Input: dimensioned drawing with shaded views. Units: mm. Origin: part minimum x, y, z. A direction names the side the tool comes from. Give positions to 0.01 mm unless a question says otherwise; leave off trailing zeros. Write each loop counter-clockwise with the first axis right and the second up, starting at its lowest first coordinate (ties: lowest second). Pieces come first, ordered by that corner, then holes. Notation, with made-up numbers: (39.25, -25.75) -> (56.25, -25.75) arc R24 cw to (56.25, -1.75) -> close; hole circle Ø10 at (70, 1.25). An arc over 180 degrees is marked (long way). Return JSON: item names as keys, results as strings. Group by question number.
Item 1: Pin query (flat end, axial travel): P1, Ø1.5, axis at x = 47.5, y = 790.5, coming from the +Z side; P2, Ø1.5, axis at y = 250.5, z = 168.5, coming from the +X side; P3, Ø8, axis at x = 73.5, y = 418.5, coming from the +Z side. Return the tip coordinate at first contact, or that it passes through.
Item 2: Section D-D, the plane z = 89. Return loops of the section in (x, y), then the cut area to 3 significant figures.
Item 3: Line query: line 1 (Z direction, x = 50, y = 231.5); line 2 (X direction, y = 511, z = 130.5) (1 decimal); line 3 (X direction, y = 529, z = 137.5). Output: solid intervals per line, ascending. Write a range as [from, to].
Item 4: Section A-A, the plane x = 50. Return loops of the section in (y, z).
Item 5: Section B-B, the plane z = 150. Return loops of the section in (x, y), then the cut area to 3 significant figures.
Item 6: Section C-C, the plane y = 500.5. Return loops of the section in (x, z), then the cut area to 3 significant figures.
Item 7: Set-up query: the marked faces 1 and 2. Return all of +Z, -Z, +X, -X, +Y, -Y with unobstructed straight access to the full face (end or side cutting, diameter ignored); none if empty.
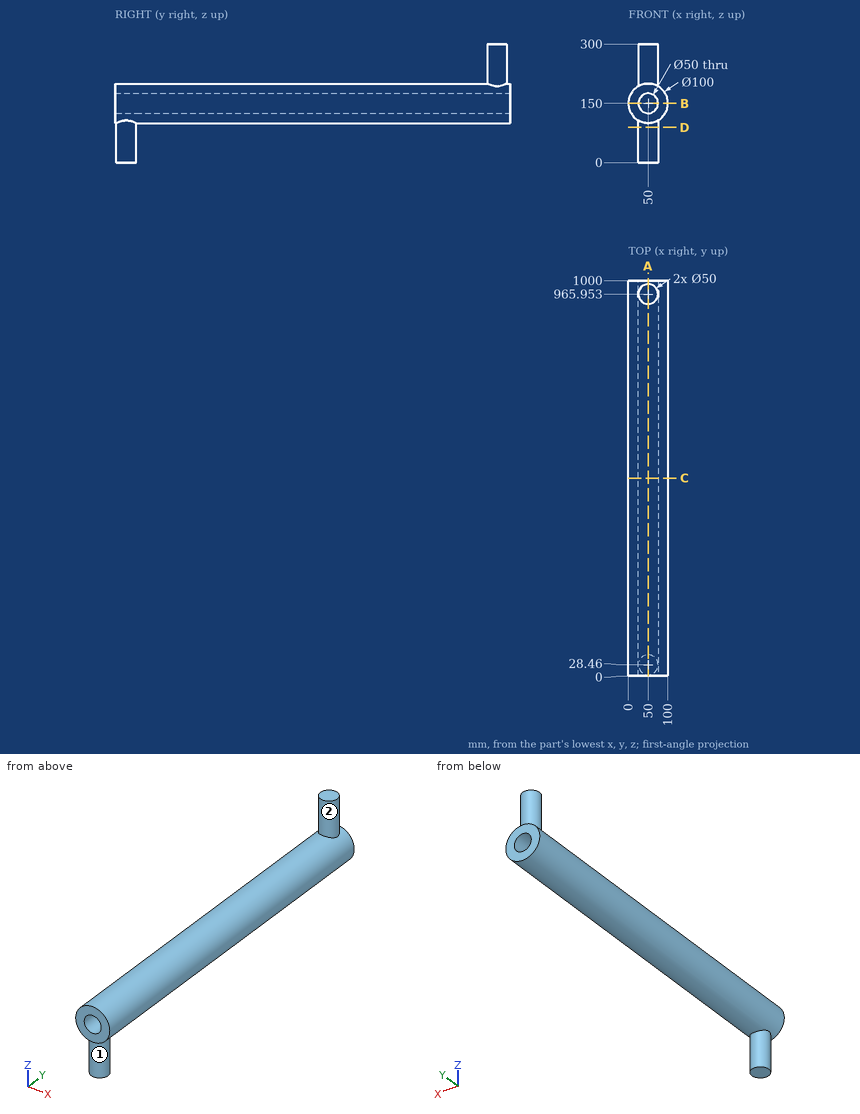
Answer below:
{
 "1": {"P1": "stops at z = 199.97", "P2": "stops at x = 96.74", "P3": "stops at z = 196.04"},
 "2": {"outline": "circle Ø50 at (50, 28.46)", "area": "1,960 mm2"},
 "3": {"line 1": "z = [100, 125], [175, 200]", "line 2": "x = [4, 34.4], [65.6, 96]", "line 3": "x = [1.59, 28.35], [71.65, 98.41]"},
 "4": {"outline": "(0, 100) -> (3.46, 100) -> (3.46, 0) -> (53.46, 0) -> (53.46, 100) -> (1000, 100) -> (1000, 125) -> (0, 125) -> close; (0, 175) -> (1000, 175) -> (1000, 200) -> (990.95, 200) -> (990.95, 300) -> (940.95, 300) -> (940.95, 200) -> (0, 200) -> close"},
 "5": {"outline": "(0, 0) -> (25, 0) -> (25, 1000) -> (0, 1000) -> close; (75, 0) -> (100, 0) -> (100, 1000) -> (75, 1000) -> close", "area": "50,000 mm2"},
 "6": {"outline": "circle Ø100 at (50, 150); hole circle Ø50 at (50, 150)", "area": "5,890 mm2"},
 "7": {"face 1": "-Z", "face 2": "+Z"}
}
